from build123d import *

# Parameters (mm, degrees)
SKETCH_1_R      = 8
SKETCH_1_R_2    = 1.5
SKETCH_1_R_3    = 1
EXTRUDE_1_DEPTH = 3


with BuildPart() as part:
    # Эскиз1 → Бобышка-Вытянуть1 (new body)
    with BuildSketch(Plane.XY):
        with BuildLine():
            Line((-22.026334366, -10.340325606), (19.973665634, -10.340325606))
            ThreePointArc((19.973665634, -10.340325606), (22.802092759, -9.168752731), (23.973665634, -6.340325606))
            Line((23.973665634, -6.340325606), (23.973665634, 4.659674394))
            ThreePointArc((23.973665634, 4.659674394), (22.802092759, 7.488101519), (19.973665634, 8.659674394))
            Line((19.973665634, 8.659674394), (-22.026334366, 8.659674394))
            Line((-22.026334366, 8.659674394), (-28.026334366, 8.659674394))
            ThreePointArc((-28.026334366, 8.659674394), (-28.733441147, 8.366781175), (-29.026334366, 7.659674394))
            Line((-29.026334366, 7.659674394), (-29.026334366, 3.659674394))
            ThreePointArc((-29.026334366, 3.659674394), (-28.733441147, 2.952567613), (-28.026334366, 2.659674394))
            Line((-28.026334366, 2.659674394), (-27.026334366, 2.659674394))
            ThreePointArc((-27.026334366, 2.659674394), (-26.319227584, 2.366781175), (-26.026334366, 1.659674394))
            Line((-26.026334366, 1.659674394), (-26.026334366, -6.340325606))
            ThreePointArc((-26.026334366, -6.340325606), (-24.85476149, -9.168752731), (-22.026334366, -10.340325606))
        make_face()
        with Locations((-1.026334366, -0.840325606)):
            Circle(SKETCH_1_R, mode=Mode.SUBTRACT)
        with Locations((-23.24262837, 5.112512431)):
            Circle(SKETCH_1_R_2, mode=Mode.SUBTRACT)
        with Locations((-11.651518455, 2.00668389)):
            Circle(SKETCH_1_R_2, mode=Mode.SUBTRACT)
        with Locations(Location((9.598849724, 2.00668389, 0), (0, 0, 180))):
            Circle(SKETCH_1_R_2, mode=Mode.SUBTRACT)
        with Locations(Location((21.189959639, 5.112512431, 0), (0, 0, 180))):
            Circle(SKETCH_1_R_2, mode=Mode.SUBTRACT)
        with Locations((-27.026334366, 5.659674394)):
            Circle(SKETCH_1_R_3, mode=Mode.SUBTRACT)
    extrude(amount=EXTRUDE_1_DEPTH)


solid = part.part
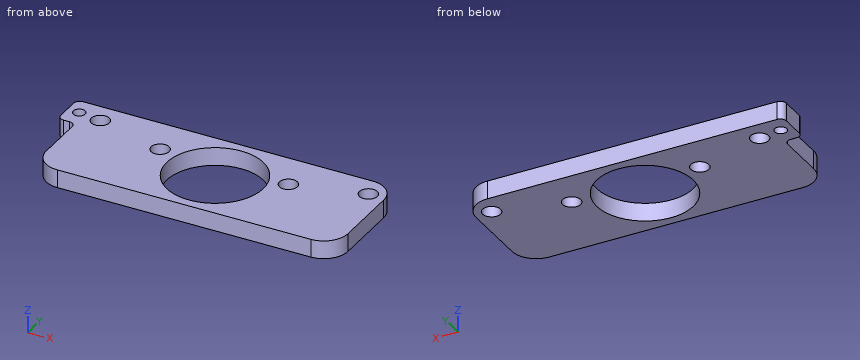
Verification items for the finished model (mm, model axes). Give positions to 0.01 mm unless a question says otherwise; leave off trailing zeros. Order: outer loops, then holes, each group sorted by start corner. A loop starts at its lowest first (then second) coordinate and runs counter-clockwise, first axis right, second up. Notation, with made-up numbers: M -21,24 L 19,24 A23 cw 19,32 Z; hole C 72.25,8 d1. An arc over 180 degrees is marked long. Use one line per item in the form item = value. Start each with the question number.
Q1. Go/stop test with flat-tipped pins: pin 1 Ø0.8 at (x, z) = (-27.5, 1.5) entering from -Y; pin 2 Ø1.5 at (y, z) = (-1, 1.5) entering from -X. Record where each tip stops, or that it passes through.
Q2. Section check B-B (x = 6). Enter the section's corners in (y, z), then the cut area to 4 significant figures.
Q3. Section check A-A (y = -4). Enter the section's corners in (x, z), then the cut area to 3 significant figures.
Q4. Scan lines: line 1 along X through (y, z) = (-1, 2.8); line 2 along Y through (x, z) = (-11.5, 1.1); line 3 along X through (y, z) = (2.75, 1). Record each from-to range of solid material in increasing order. Write a range as [from, to].
Q5. Section check C-C (z = 0.85). Enter the section's corners in (x, y), then the cut area to 3 significant figures.
Evaluation:
q1.pin_1 = 2.66
q1.pin_2 = -26.03
q2.outline = M -10.34,0 L -4.67,0 L -4.67,3 L -10.34,3 Z; M 2.98,0 L 8.66,0 L 8.66,3 L 2.98,3 Z
q2.area = 34.05 mm2
q3.outline = M -26.03,0 L -8.38,0 L -8.38,3 L -26.03,3 Z; M 6.32,0 L 23.97,0 L 23.97,3 L 6.32,3 Z
q3.area = 106 mm2
q4.line_1 = [-26.03, -9.02], [6.97, 23.97]
q4.line_2 = [-10.34, 0.51], [3.5, 8.66]
q4.line_3 = [-28.44, -12.95], [-10.35, -8.18], [6.12, 8.3], [10.9, 23.97]
q5.outline = M -29.03,3.66 A1 ccw -28.03,2.66 L -27.03,2.66 A1 cw -26.03,1.66 L -26.03,-6.34 A4 ccw -22.03,-10.34 L 19.97,-10.34 A4 ccw 23.97,-6.34 L 23.97,4.66 A4 ccw 19.97,8.66 L -28.03,8.66 A1 ccw -29.03,7.66 Z; hole C -27.03,5.66 d2; hole C -23.24,5.11 d3; hole C -11.65,2.01 d3; hole C -1.03,-0.84 d16; hole C 9.6,2.01 d3; hole C 21.19,5.11 d3
q5.area = 725 mm2
